Geometry check sheet. Reference: drawing and pictorial views, mm from the part's lowest x, y, z. A direction names the side the tool comes from. Give positions to 0.01 mm unless a question says otherwise; leave off trailing zeros. Order: outer loops, then holes, each group sorted by start corner. A loop starts at its lowest first (then second) coordinate and runs counter-clockwise, first axis right, second up.
Item 1: Sectioned sample at B-B on y = 5.5. Record the boundary of the cut face in (x, z).
Item 2: Sectioned sample at A-A on x = 10.75. Record the boundary of the cut face in (y, z) (3 decimals), and give its area (3 significant figures).
Item 3: Material ranges on line 1 along Y through (x, z) = (10.75, 1.55) (3 decimals); line 2 along X through (y, z) = (4.5, 3); line 3 along X through (y, z) = (20, 0.7), recorded low to high.
Item 4: Sectioned sample at C-C on z = 0.55. Record the boundary of the cut face in (x, y) (3 decimals).
Item 5: Release check for a two-part mould opening along Y. For the marked faces 3, 4 and 5 record: released by +Y, released by -Y, zero draft, split by the parting line, or undercut.
Item 6: Access from +Z, -Z, +X, -X, +Y, -Y to the whole of each face (thin tool, end or side, straight path). Record for the marked faces 1 and 2.
Item 7: Gauge pin test, flat ends, axial feed: P1, Ø1.6, axis at x = 1.5, z = 2, coming from the -Y side; P2, Ø4, axis at x = 10.75, y = 18.075, coming from the -Z side. Record the tip position at first contact, or that the pin passes through.
Item 8: Sectioned sample at D-D on x = 2.5. Record the boundary of the cut face in (y, z), and give its area (3 significant figures).
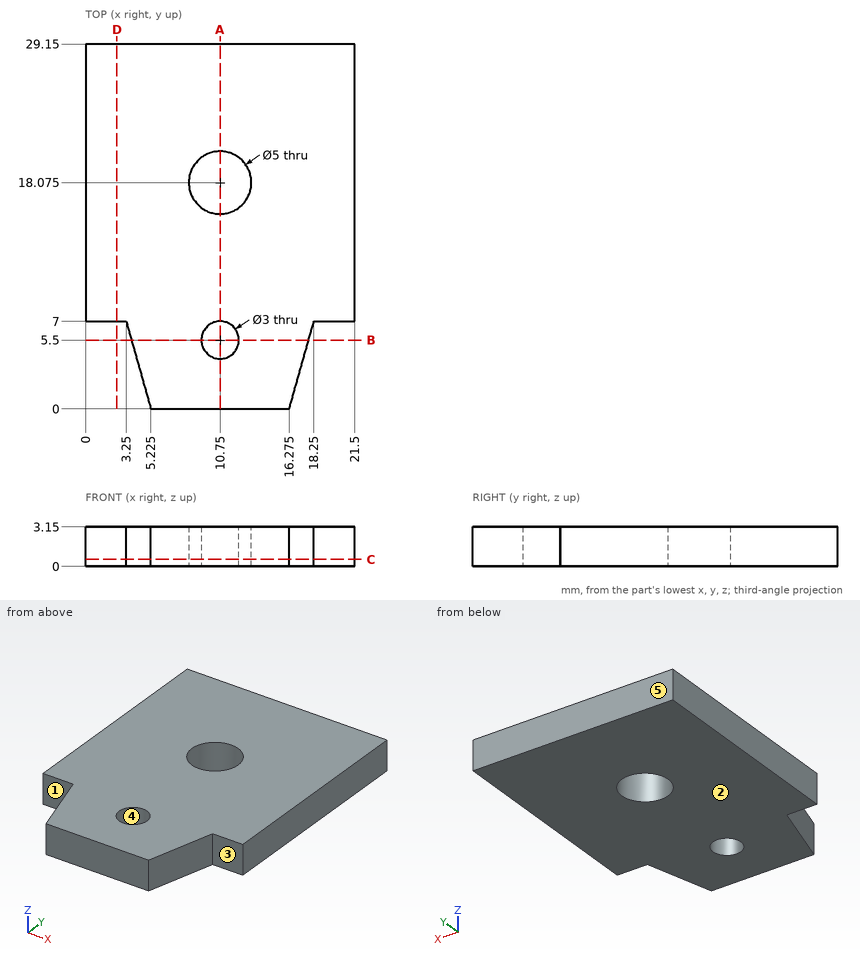
Report:
1. outline: (3.67, 0) - (9.25, 0) - (9.25, 3.15) - (3.67, 3.15) - close; (12.25, 0) - (17.83, 0) - (17.83, 3.15) - (12.25, 3.15) - close
2. outline: (0, 0) - (4, 0) - (4, 3.15) - (0, 3.15) - close; (7, 0) - (15.575, 0) - (15.575, 3.15) - (7, 3.15) - close; (20.575, 0) - (29.15, 0) - (29.15, 3.15) - (20.575, 3.15) - close
2. area: 66.6 mm2
3. line 1: y = 0 to 4, 7 to 15.575, 20.575 to 29.15
3. line 2: x = 3.96 to 9.63, 11.87 to 17.54
3. line 3: x = 0 to 9.15, 12.35 to 21.5
4. outline: (0, 7) - (3.25, 7) - (5.225, 0) - (16.275, 0) - (18.25, 7) - (21.5, 7) - (21.5, 29.15) - (0, 29.15) - close; hole circle Ø5 at (10.75, 18.075); hole circle Ø3 at (10.75, 5.5)
5. face 3: released by -Y
5. face 4: undercut
5. face 5: released by +Y
6. face 1: +Z, -Z, -X, -Y
6. face 2: -Z, +X, -X, +Y, -Y
7. P1: stops at y = 7
7. P2: passes through
8. outline: (7, 0) - (29.15, 0) - (29.15, 3.15) - (7, 3.15) - close
8. area: 69.8 mm2
